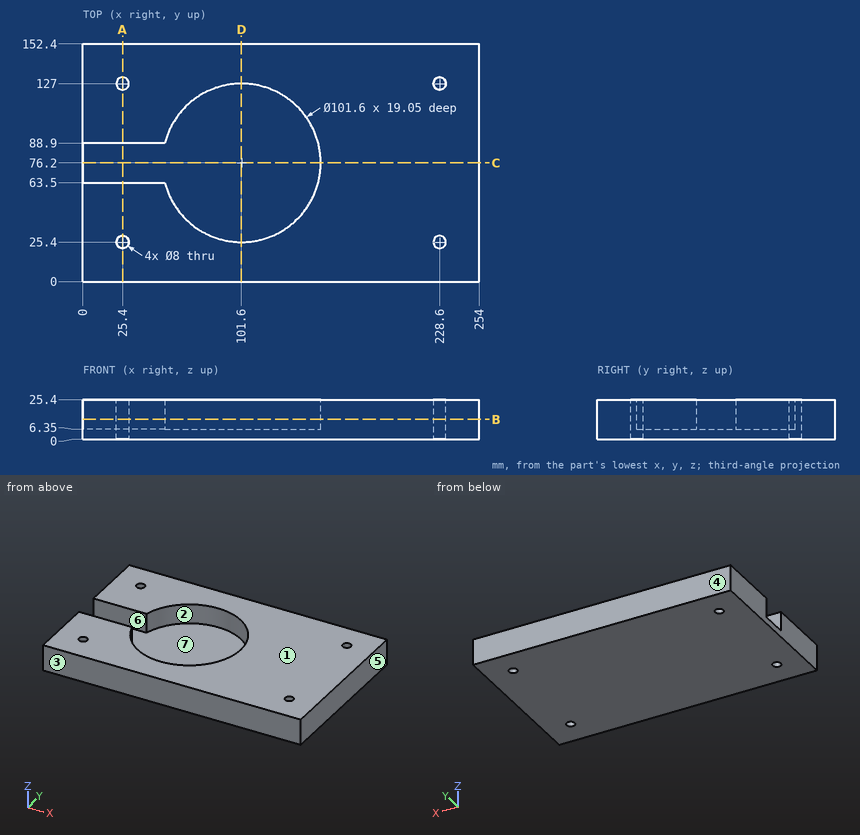
For this review, use the dimensioned drawing (mm, ordinates from the lowest corner) and the shaded views. A direction names the side the tool comes from. Coordinates: 2 decimals unless noted, no trailing zeros. Write each loop counter-clockwise with the first axis right and the second up, starting at its lowest first coordinate (ties: lowest second). Pieces come first, ordered by that corner, then holes. Notation, with made-up numbers: (32, 6.25) - (51, 6.25) arc R16 cw to (51, 29.25) - close; hole circle Ø2 at (32.5, 16). An arc over 180 degrees is marked (long way). Answer as a JSON object with one key per item and string values. Group by question number.
1. Add section D-D (x = 101.6). Give the boundary of the cut face in (y, z).
2. Clearance check with flat-ended pins moving along their axes: pin 1 Ø6.5 at (x, y) = (228.6, 25.4) entering from +Z; pin 2 Ø4 at (x, y) = (146.5, 70.5) entering from +Z. State where each tip first meets the part, or that it passes through.
3. Add section A-A (x = 25.4). Give the boundary of the cut face in (y, z).
4. Machinability: for the marked faces 5, 6 and 7, which of the approach directions +Z, -Z, +X, -X, +Y, -Y give a long, thin tool a straight path to every point of the face, cutting with its end or side? Answer none if there is none.
5. Add section B-B (z = 12.75). Give the boundary of the cut face in (x, y), plus the area to 3 significant figures.
6. To check wall thickness, follow probe 1 along Y at (x, z) = (228.6, 9); probe 2 along Y at (x, z) = (16, 21); probe 3 along Y at (x, z) = (25.4, 12.75). State the ranges of each line that lie inside material, in increasing order.
7. Mouldability with a two-part tool opening along Y and no side actions: class the marked faces 1, 2, 3 and 4 as pulls with the +Y half, pulls with the -Y half, needs draft (parallel to the pull), parting line crosses it, or undercut.
8. Add section C-C (y = 76.2). Give the boundary of the cut face in (x, z).
Findings:
{
 "1": {"outline": "(0, 0) - (152.4, 0) - (152.4, 25.4) - (127, 25.4) - (127, 6.35) - (25.4, 6.35) - (25.4, 25.4) - (0, 25.4) - close"},
 "2": {"pin 1": "through", "pin 2": "z = 6.35"},
 "3": {"outline": "(0, 0) - (21.4, 0) - (21.4, 25.4) - (0, 25.4) - close; (29.4, 0) - (123, 0) - (123, 25.4) - (88.9, 25.4) - (88.9, 6.35) - (63.5, 6.35) - (63.5, 25.4) - (29.4, 25.4) - close; (131, 0) - (152.4, 0) - (152.4, 25.4) - (131, 25.4) - close"},
 "4": {"face 5": "+Z, -Z, +X, +Y, -Y", "face 6": "+Z, -X", "face 7": "+Z"},
 "5": {"outline": "(0, 0) - (254, 0) - (254, 152.4) - (0, 152.4) - (0, 88.9) - (52.41, 88.9) arc R50.8 cw (long way) to (52.41, 63.5) - (0, 63.5) - close; hole circle Ø8 at (25.4, 25.4); hole circle Ø8 at (25.4, 127); hole circle Ø8 at (228.6, 25.4); hole circle Ø8 at (228.6, 127)", "area": "29,100 mm²"},
 "6": {"probe 1": "0 to 21.4, 29.4 to 123, 131 to 152.4", "probe 2": "0 to 63.5, 88.9 to 152.4", "probe 3": "0 to 21.4, 29.4 to 63.5, 88.9 to 123, 131 to 152.4"},
 "7": {"face 1": "needs draft", "face 2": "undercut", "face 3": "pulls with the -Y half", "face 4": "pulls with the +Y half"},
 "8": {"outline": "(0, 0) - (254, 0) - (254, 25.4) - (152.4, 25.4) - (152.4, 6.35) - (0, 6.35) - close"}
}
